The listing builds one solid part. Answer for the finished solid, in the listing's coordinates (mm). Round coordinates to 2 decimals unless told otherwise and drop trailing zeros. Write each loop counter-clockwise with the first axis right and the second up, starting at its lowest first coordinate (ties: lowest second). Pieces come first, ordered by that corner, then holes.
(1) Find the intervals of material crossed by probe 1 along X at (y, z) = (1, 42); probe 2 along Y at (x, z) = (0, 22); probe 3 along X at (y, z) = (-13.5, 11.5), in increasing order.
(2) A cutting plane is placed at A-A, the plane x = 0. Give the vertices of the cut face in (y, z).
(3) The mould has two halves that part along Y. Classify faces 1 (the face through (14, 25, 53.34)), 2 (the face through (-3.023, 23.026, 26.972)), 3 (the face through (-8.25, -37.14, 26.37)): +Y half, -Y half, draft (parallel to the pull), parting line (faces both ways), or undercut.
(4) Each of these flat-tipped pins is pushed along its axis until it touches: pin 1 Ø1 at (y, z) = (15.5, 20.5) entering from +X; pin 2 Ø4 at (x, z) = (-18.5, 35) entering from -Y; pin 3 Ø4 at (y, z) = (-7, 19.5) entering from -X; pin 4 Ø6 at (x, y) = (-17.5, 3.5) entering from +Z. Where does it stop, or does it pass through?
(5) A cutting plane is placed at C-C, the plane z = 23. Give the vertices of the cut face in (x, y), and give its area (3 significant figures).
from build123d import *

# Parameters (mm, degrees)
F0_R     = 38.043334
F1_DEPTH = 53.34
F2_R     = 23.223229
F3_DEPTH = 53.34
F4_R     = 5.08


with BuildPart() as f1:
    # F0 (on Top) → F1 (new body)
    with BuildSketch(Plane.XY):
        Circle(F0_R)
    extrude(amount=F1_DEPTH)

    # F2 (on face) → F3 (cut, through all)
    with BuildSketch(Plane.XY.offset(53.34)):
        Circle(F2_R)
    extrude(amount=-F3_DEPTH, mode=Mode.SUBTRACT)

    # F4
    f4_edges = [f1.edges().sort_by_distance(p)[0] for p in [
        (-38.043334, 0, 53.34),
        (-23.223229, 0, 53.34),
        (-38.043334, 0, 0),
        (-23.223229, 0, 0),
    ]]
    fillet(f4_edges, radius=F4_R)


solid = f1.part
Solutions:
1. probe 1: x = -38.03 to -23.2, 23.2 to 38.03
1. probe 2: y = -38.04 to -23.22, 23.22 to 38.04
1. probe 3: x = -35.57 to -18.9, 18.9 to 35.57
2. outline: (-38.04, 5.08) arc R5.08 ccw to (-32.96, 0) - (-28.3, 0) arc R5.08 ccw to (-23.22, 5.08) - (-23.22, 48.26) arc R5.08 ccw to (-28.3, 53.34) - (-32.96, 53.34) arc R5.08 ccw to (-38.04, 48.26) - close; (23.22, 5.08) arc R5.08 ccw to (28.3, 0) - (32.96, 0) arc R5.08 ccw to (38.04, 5.08) - (38.04, 48.26) arc R5.08 ccw to (32.96, 53.34) - (28.3, 53.34) arc R5.08 ccw to (23.22, 48.26) - close
3. face 1: draft
3. face 2: undercut
3. face 3: parting line
4. pin 1: stops at x = 34.96
4. pin 2: stops at y = -34.28
4. pin 3: stops at x = -37.71
4. pin 4: passes through
5. outline: circle Ø76.09 at (0, 0); hole circle Ø46.45 at (0, 0)
5. area: 2,850 mm2
